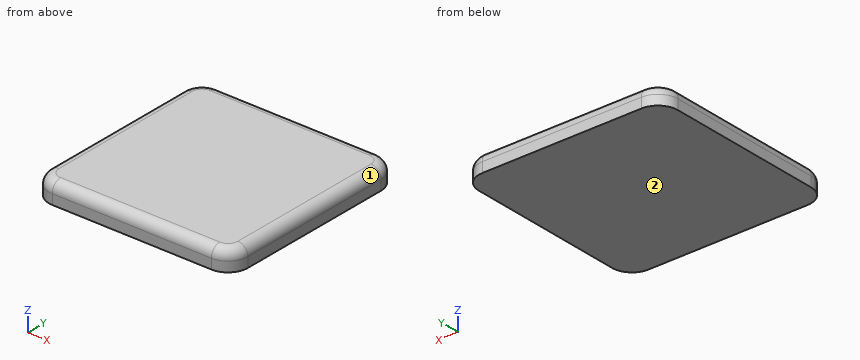
Autodesk Inventor part; units mm, degrees
ref_plane "YZ Plane" through (0, 0, 0) normal (1, 0, 0) x (0, 1, 0)
ref_plane "XZ Plane" through (0, 0, 0) normal (0, 1, 0) x (-1, 0, 0)
ref_plane "XY Plane" through (0, 0, 0) normal (0, 0, 1) x (1, 0, 0)
sketch "Skizze1" plane through (0, 0, 0) normal (0, 0, 1) x (1, 0, 0)
  line L0 (-20, 20) -> (20, 20)
  line L1 (20, 20) -> (20, -20)
  line L2 (20, -20) -> (-20, -20)
  line L3 (-20, -20) -> (-20, 20)
  line L4 (-20, 20) -> (20, -20) construction
  line L5 (20, 20) -> (-20, -20) construction
  point P0 (0, 0)
  dimension "d0" = 40
  dimension "d1" = 40
extrude "Extrusion1" add sketch "Skizze1" along normal blind 4
fillet "Rundung1" radius 4 4 edges at (-20, -20, 2) (20, -20, 2) (-20, 20, 2) (20, 20, 2)
fillet "Rundung2" radius 2 8 edges at (18.8284, -18.8284, 4) (20, 0, 4) (18.8284, 18.8284, 4) (0, 20, 4) (-18.8284, 18.8284, 4) (-20, 0, 4) (-18.8284, -18.8284, 4) (0, -20, 4)
properties part number "Abdeckkappe-40x40x4"
Geometry check sheet. Reference: the model listing, model coordinates, mm. Face numbers are marked on the shaded views. Round coordinates to 2 decimals unless told otherwise and drop trailing zeros. Answer as CSV lines item,"result".
1) Thickness scan on probe 1 along X at (y, z) = (-2, 2.4); probe 2 along Z at (x, y) = (-17.5, 18); probe 3 along Y at (x, z) = (-12.5, 3.25). Record the ranges inside material, lowest first. Write a range as [from, to].
Entries:
probe 1,"[-19.96, 19.96]"
probe 2,"[0, 3.94]"
probe 3,"[-19.56, 19.56]"
2) Mould release check, pull along Z, two halves, no side actions. Record for the marked faces 1 and 2: +Z half, -Z half, draft (parallel to the pull), parting line (faces both ways), or undercut.
Entries:
face 1,"+Z half"
face 2,"-Z half"
3) Gauge pin test, flat end, axial feed: pin 1 Ø8 at (x, y) = (13.5, -0.5) entering from -Z. Record the tip position at first contact, or that the pin passes through.
Entries:
pin 1,"z = 0"
